from build123d import *

# Parameters (mm, degrees)
F0_W         = 66
F0_H         = 26
F0_W_2       = 60
F0_H_2       = 20
F1_DEPTH     = 70
F2_R         = 4
F3_DEPTH     = 25
F4_T1_DEPTH  = 60
F4_T3_DEPTH  = 20
F4_T9_DEPTH  = 72.8584149398
F4_T15_DEPTH = 32.8584149398
F4_T24_DEPTH = 72.8584149398
F4_T30_DEPTH = 32.8584149398
F4_T39_DEPTH = 72.8584149398
F4_T45_DEPTH = 32.8584149398
F4_T54_DEPTH = 32.8584149398
F4_T60_DEPTH = 72.8584149398
F5_T1_DEPTH  = 91.7168298797


# Not quite as in the source:
# - a fillet or chamfer that OpenCascade refuses, or shapes differently, is made with other operations: its cross-section is extruded or revolved along the edge and cut away or added


with BuildPart() as f1:
    # F0 (on Front) → F1 (new body)
    with BuildSketch(Plane.XZ):
        with Locations((1.3007868016, 6.4724322181)):
            Rectangle(F0_W, F0_H)
        with Locations((1.3007868016, 6.4724322181)):
            Rectangle(F0_W_2, F0_H_2, mode=Mode.SUBTRACT)
    extrude(amount=F1_DEPTH)

    # F2 (on face) → F3 (join)
    with BuildSketch(Plane.YZ.offset(34.3007868016)):
        with Locations((-60, 4.4724322181)):
            Circle(F2_R)
        with Locations((-10, 4.4724322181)):
            Circle(F2_R)
    extrude(amount=F3_DEPTH)

    # F4: chamfer of 5 on 4 edges, made by hand

    # F4_s2 → F4_t1 (cut)
    with BuildSketch(Plane.YZ.offset(-28.6992131984)):
        Polygon((-70, 21.4724322181), (-65, 16.4724322181), (-70, 16.4724322181), align=None)
        Polygon((-70, -8.5275677819), (-65, -3.5275677819), (-70, -3.5275677819), align=None)
    extrude(amount=F4_T1_DEPTH, mode=Mode.SUBTRACT)

    # F4_s4 → F4_t3 (cut)
    with BuildSketch(Plane.XY.offset(-3.5275677819)):
        Polygon((-33.6992131984, -70), (-28.6992131984, -65), (-28.6992131984, -70), align=None)
        Polygon((36.3007868016, -70), (31.3007868016, -65), (31.3007868016, -70), align=None)
    extrude(amount=F4_T3_DEPTH, mode=Mode.SUBTRACT)


with BuildPart() as f4_tool7:
    # F4_s8 → F4_t9 (new body)
    with BuildSketch(Plane.YZ.offset(-41.5576281383)):
        Polygon((-70, 21.4724322181), (-65, 16.4724322181), (-70, 16.4724322181), align=None)
    extrude(amount=F4_T9_DEPTH)

    split(bisect_by=Plane.YZ.offset(-31.6992131984), keep=Keep.TOP)

    split(bisect_by=Plane.XY.offset(19.4724322181), keep=Keep.BOTTOM)

    split(bisect_by=Plane.YZ.offset(-28.6992131984), keep=Keep.BOTTOM)


with BuildPart() as f4_tool13:
    # F4_s14 → F4_t15 (new body)
    with BuildSketch(Plane.XY.offset(-3.5275677819)):
        Polygon((-33.6992131984, -70), (-28.6992131984, -65), (-28.6992131984, -70), align=None)
    extrude(amount=F4_T15_DEPTH)

    split(bisect_by=Plane.YZ.offset(-31.6992131984), keep=Keep.TOP)

    split(bisect_by=Plane.XY.offset(19.4724322181), keep=Keep.BOTTOM)

    split(bisect_by=Plane.XY.offset(16.4724322181), keep=Keep.TOP)


with BuildPart() as f4_tool7_1:
    add(f4_tool7.part)

    # F4_t19: intersect F4_tool13
    add(f4_tool13.part, mode=Mode.INTERSECT)


with BuildPart() as f1_1:
    add(f1.part)

    # F4_t5: cut F4_tool7
    add(f4_tool7_1.part, mode=Mode.SUBTRACT)


with BuildPart() as f4_tool22:
    # F4_s23 → F4_t24 (new body)
    with BuildSketch(Plane.YZ.offset(-28.6992131984)):
        Polygon((-70, 21.4724322181), (-65, 16.4724322181), (-70, 16.4724322181), align=None)
    extrude(amount=F4_T24_DEPTH)

    split(bisect_by=Plane.YZ.offset(34.3007868016), keep=Keep.BOTTOM)

    split(bisect_by=Plane.XY.offset(19.4724322181), keep=Keep.BOTTOM)

    split(bisect_by=Plane.YZ.offset(31.3007868016), keep=Keep.TOP)


with BuildPart() as f4_tool28:
    # F4_s29 → F4_t30 (new body)
    with BuildSketch(Plane.XY.offset(29.3308471579)):
        Polygon((36.3007868016, -70), (31.3007868016, -65), (31.3007868016, -70), align=None)
    extrude(amount=-F4_T30_DEPTH)

    split(bisect_by=Plane.YZ.offset(34.3007868016), keep=Keep.BOTTOM)

    split(bisect_by=Plane.XY.offset(19.4724322181), keep=Keep.BOTTOM)

    split(bisect_by=Plane.XY.offset(16.4724322181), keep=Keep.TOP)


with BuildPart() as f4_tool22_1:
    add(f4_tool22.part)

    # F4_t34: intersect F4_tool28
    add(f4_tool28.part, mode=Mode.INTERSECT)


with BuildPart() as f1_2:
    add(f1_1.part)

    # F4_t20: cut F4_tool22
    add(f4_tool22_1.part, mode=Mode.SUBTRACT)


with BuildPart() as f4_tool37:
    # F4_s38 → F4_t39 (new body)
    with BuildSketch(Plane.YZ.offset(31.3007868016)):
        Polygon((-70, -8.5275677819), (-65, -3.5275677819), (-70, -3.5275677819), align=None)
    extrude(amount=-F4_T39_DEPTH)

    split(bisect_by=Plane.XY.offset(-6.5275677819), keep=Keep.TOP)

    split(bisect_by=Plane.YZ.offset(-31.6992131984), keep=Keep.TOP)

    split(bisect_by=Plane.YZ.offset(-28.6992131984), keep=Keep.BOTTOM)


with BuildPart() as f4_tool43:
    # F4_s44 → F4_t45 (new body)
    with BuildSketch(Plane.XY.offset(-16.3859827218)):
        Polygon((-33.6992131984, -70), (-28.6992131984, -65), (-28.6992131984, -70), align=None)
    extrude(amount=F4_T45_DEPTH)

    split(bisect_by=Plane.XY.offset(-6.5275677819), keep=Keep.TOP)

    split(bisect_by=Plane.YZ.offset(-31.6992131984), keep=Keep.TOP)

    split(bisect_by=Plane.XY.offset(-3.5275677819), keep=Keep.BOTTOM)


with BuildPart() as f4_tool37_1:
    add(f4_tool37.part)

    # F4_t49: intersect F4_tool43
    add(f4_tool43.part, mode=Mode.INTERSECT)


with BuildPart() as f1_3:
    add(f1_2.part)

    # F4_t35: cut F4_tool37
    add(f4_tool37_1.part, mode=Mode.SUBTRACT)


with BuildPart() as f4_tool52:
    # F4_s53 → F4_t54 (new body)
    with BuildSketch(Plane.XY.offset(16.4724322181)):
        Polygon((36.3007868016, -70), (31.3007868016, -65), (31.3007868016, -70), align=None)
    extrude(amount=-F4_T54_DEPTH)

    split(bisect_by=Plane.XY.offset(-6.5275677819), keep=Keep.TOP)

    split(bisect_by=Plane.YZ.offset(34.3007868016), keep=Keep.BOTTOM)

    split(bisect_by=Plane.XY.offset(-3.5275677819), keep=Keep.BOTTOM)


with BuildPart() as f4_tool58:
    # F4_s59 → F4_t60 (new body)
    with BuildSketch(Plane.YZ.offset(44.1592017414)):
        Polygon((-70, -8.5275677819), (-65, -3.5275677819), (-70, -3.5275677819), align=None)
    extrude(amount=-F4_T60_DEPTH)

    split(bisect_by=Plane.XY.offset(-6.5275677819), keep=Keep.TOP)

    split(bisect_by=Plane.YZ.offset(34.3007868016), keep=Keep.BOTTOM)

    split(bisect_by=Plane.YZ.offset(31.3007868016), keep=Keep.TOP)


with BuildPart() as f4_tool52_1:
    add(f4_tool52.part)

    # F4_t64: intersect F4_tool58
    add(f4_tool58.part, mode=Mode.INTERSECT)


with BuildPart() as f1_4:
    add(f1_3.part)

    # F4_t50: cut F4_tool52
    add(f4_tool52_1.part, mode=Mode.SUBTRACT)

    # F5: chamfer of 5 on 1 edges, made by hand

    # F5_s2 → F5_t1 (cut)
    with BuildSketch(Plane.YZ.offset(-44.5576281383)):
        Polygon((-5, 19.4724322181), (0, 14.4724322181), (0, 19.4724322181), align=None)
    extrude(amount=F5_T1_DEPTH, mode=Mode.SUBTRACT)


solid = f1_4.part
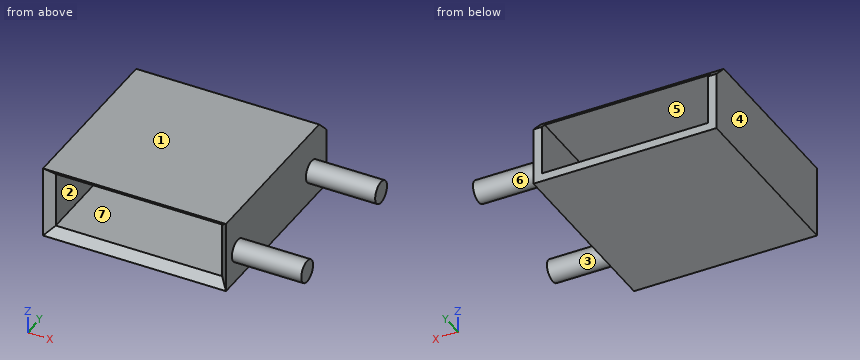
CAD build for the part. Positions are in the model's coordinates, mm. Face numbers are marked on the shaded views. A direction names the side the tool comes from. Round coordinates to 2 decimals unless told otherwise and drop trailing zeros. Loops run counter-clockwise (first coordinate to the right, second up) from the corner with the lowest first, then second, coordinate; pieces in that order, holes last. Notation, with made-up numbers: (-32.5, 55) - (4.5, 55) arc R26 ccw to (4.5, 76) - close; hole circle Ø1 at (30.5, -25). An arc over 180 degrees is marked (long way). Put each result on its own line as item: value.
1. 3-axis set-ups, long thin cutter, end or side, ignore diameter. For the marked faces 1, 2 and 3: which of +Z, -Z, +X, -X, +Y, -Y reach the whole face in a straight line?
Geometry check:
face 1: +Z, +X, -X, +Y, -Y
face 2: +Y, -Y
face 3: +X
2. Wall check: line 1 (X direction, y = -47.5, z = 0.25); line 2 (Z direction, x = -21, y = -51.5); line 3 (X direction, y = -62.5, z = 2.5). Give the ranges that are in metal, low to high.
Geometry check:
line 1: -31.7 to -28.7, 31.3 to 34.3
line 2: -6.53 to -3.53, 16.47 to 19.47
line 3: -31.7 to -28.7, 31.3 to 59.3
3. Slice it at B-B on y = -10. List the corners of the cut face in (x, z), and give its area (3 significant figures).
Geometry check:
outline: (-31.7, -6.53) - (34.3, -6.53) - (34.3, 0.47) - (59.3, 0.47) - (59.3, 8.47) - (34.3, 8.47) - (34.3, 19.47) - (-31.7, 19.47) - close; hole (-28.7, -3.53) - (31.3, -3.53) - (31.3, 16.47) - (-28.7, 16.47) - close
area: 716 mm²
4. Two-plate mould, pull along X, no slides. Class the marked faces 4, 5, 6 and 7: released by +X, released by -X, zero draft, split by the parting line, or undercut.
Geometry check:
face 4: released by -X
face 5: undercut
face 6: zero draft
face 7: undercut
5. Slice it at C-C on y = -22.5. List the corners of the cut face in (x, z).
Geometry check:
outline: (-31.7, -6.53) - (34.3, -6.53) - (34.3, 19.47) - (-31.7, 19.47) - close; hole (-28.7, -3.53) - (31.3, -3.53) - (31.3, 16.47) - (-28.7, 16.47) - close
6. Slice it at D-D on x = 47. List the corners of the cut face in (y, z), and give its area (3 significant figures).
Geometry check:
outline: circle Ø8 at (-60, 4.47); circle Ø8 at (-10, 4.47)
area: 101 mm²
7. Pin check, flat tips, straight feed: P1, Ø1.5, axis at x = 44.5, y = -59.5, coming from the +Z side; P2, Ø5, axis at x = 49, z = 0.5, coming from the -Y side; P3, Ø6, axis at y = -18.5, z = 11, coming from the +X side. Stop position of each tip, or through.
Geometry check:
P1: z = 8.47
P2: y = -63.72
P3: x = 34.3
8. Slice it at A-A on x = 21. List the corners of the cut face in (y, z), and give its area (4 significant figures).
Geometry check:
outline: (-68, -6.53) - (0, -6.53) - (0, -3.53) - (-65, -3.53) - close; (-68, 19.47) - (-65, 16.47) - (-2, 16.47) - (-5, 19.47) - close
area: 388.5 mm²
